Source: three-view drawing plus pictorial views. Frame: mm from the lowest corner of the part. Give positions to 0.01 mm unless a question says otherwise; leave off trailing zeros. Loops run counter-clockwise (first coordinate to the right, second up) from the corner with the lowest first, then second, coordinate; pieces in that order, holes last. Notation, with made-up numbers: (60, -14.5) - (66, -14.5) arc R21 ccw to (66, -0.5) - close; hole circle Ø9 at (60, 14.5). An arc over 180 degrees is marked (long way). Answer as a JSON object with one key per item and string values.
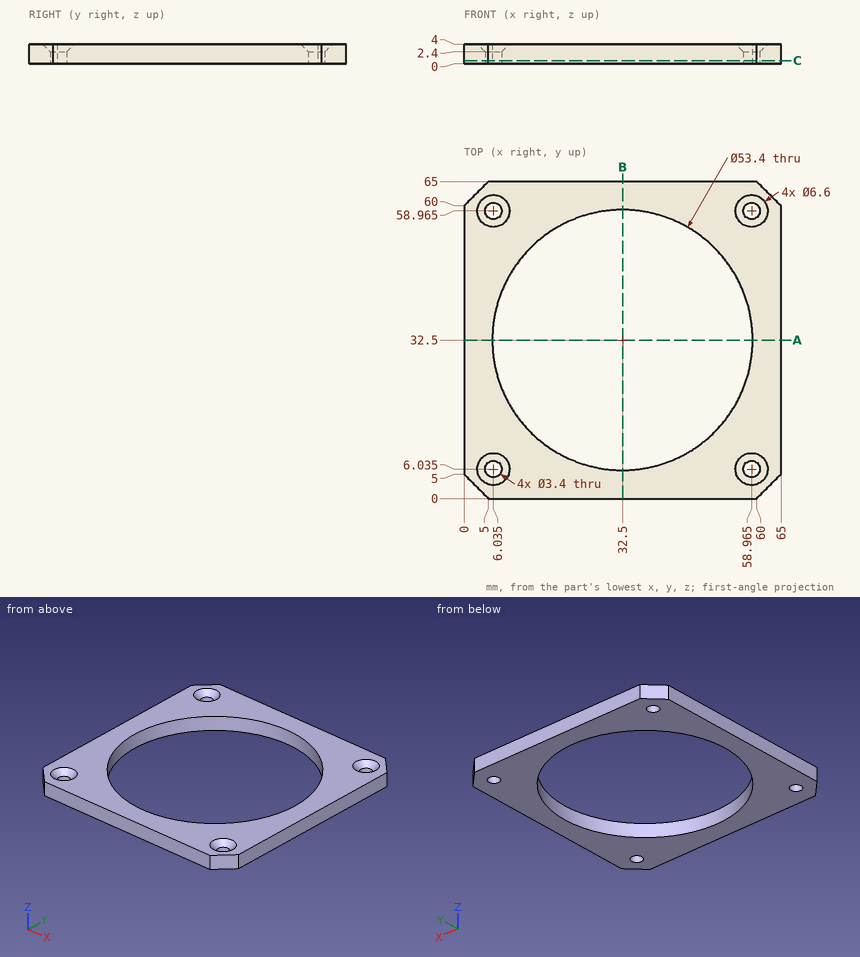
Item 1: Cut plane C-C (z = 0.6). Return loops of the section in (x, y) (1 decimal).
Geometry check:
{"outline": "(0, 5) - (5, 0) - (60, 0) - (65, 5) - (65, 60) - (60, 65) - (5, 65) - (0, 60) - close; hole circle Ø3.4 at (6, 6); hole circle Ø3.4 at (6, 59); hole circle Ø53.4 at (32.5, 32.5); hole circle Ø3.4 at (59, 6); hole circle Ø3.4 at (59, 59)"}
Item 2: Material intervals for line 1 (Y direction, x = 32.5, z = 2.25); line 2 (Y direction, x = 9.5, z = 2.05) (1 decimal); line 3 (X direction, y = 27, z = 1.7), sorted ascending. Write a range as [from, to].
Geometry check:
{"line 1": "y = [0, 5.8], [59.2, 65]", "line 2": "y = [0, 18.9], [46.1, 65]", "line 3": "x = [0, 6.37], [58.63, 65]"}
Item 3: Contact query for a flat-ended pin moving along its axis: P1, Ø2, axis at x = 6.04, y = 6.04, coming from the +Z side. Output: stop coordinate, or through.
Geometry check:
{"P1": "passes through"}
Item 4: Cut plane A-A (y = 32.5). Return loops of the section in (x, z).
Geometry check:
{"outline": "(0, 0) - (5.8, 0) - (5.8, 4) - (0, 4) - close; (59.2, 0) - (65, 0) - (65, 4) - (59.2, 4) - close"}
